Check sheet for the drawn part. Datum: minimum x, y, z corner. Units: mm. A direction names the side the tool comes from. Round coordinates to 2 decimals unless told otherwise and drop trailing zeros. Write each loop counter-clockwise with the first axis right and the second up, starting at its lowest first coordinate (ties: lowest second). Pieces come first, ordered by that corner, then holes.
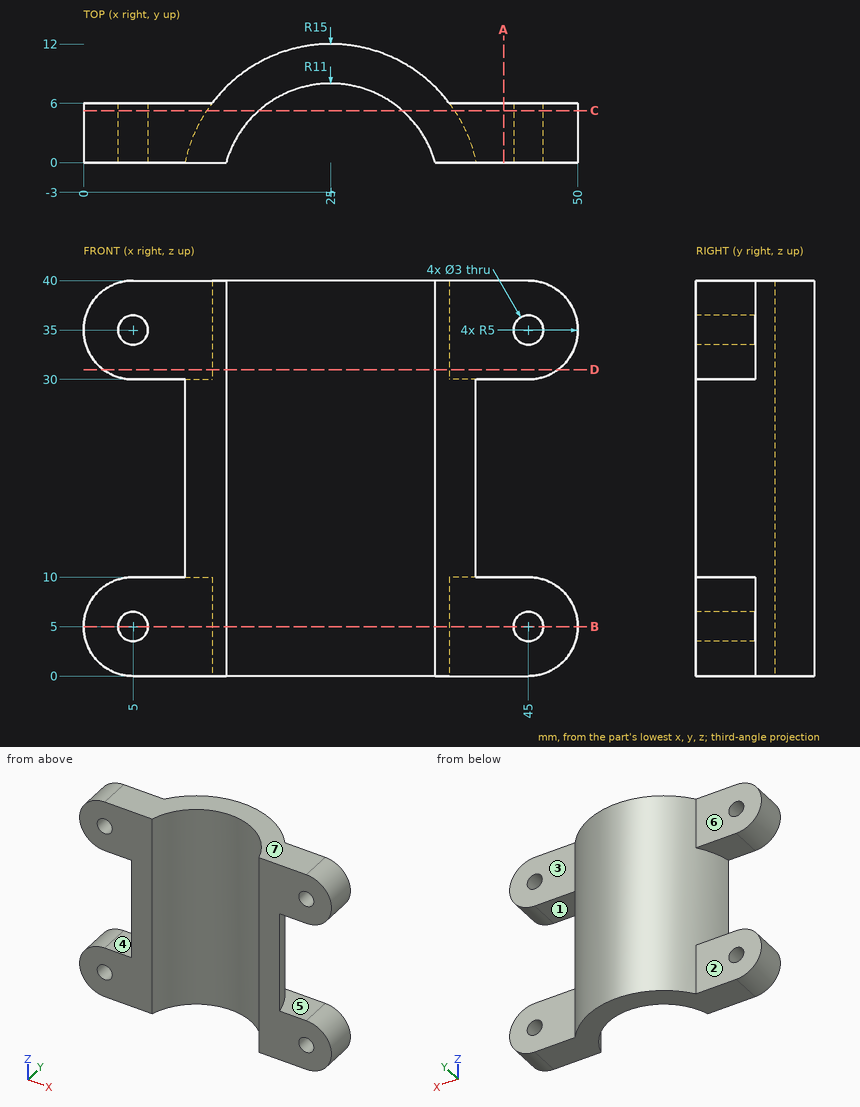
Q1. Depth check by flat-ended pin: P1, Ø4, axis at x = 45, z = 5, coming from the +Y side; P2, Ø1.8, axis at x = 5, z = 35, coming from the +Y side; P3, Ø1, axis at y = 10, z = 6.5, coming from the -X side. Enter the tip coordinate at first touch or a pass-through.
Recorded:
P1: stops at y = 6
P2: passes through
P3: stops at x = 16.71
Q2. Sectioned sample at B-B (z = 5). Enter the section's corners in (x, y).
Recorded:
outline: (0, 0) - (3.5, 0) - (3.5, 6) - (0, 6) - close; (6.5, 0) - (14.42, 0) arc R11 cw to (35.58, 0) - (43.5, 0) - (43.5, 6) - (37, 6) arc R15 ccw to (13, 6) - (6.5, 6) - close; (46.5, 0) - (50, 0) - (50, 6) - (46.5, 6) - close
Q3. Release check for a two-part mould opening along Z. For the marked faces 5, 6 and 7 record: released by +Z, released by -Z, zero draft, split by the parting line, or undercut.
Recorded:
face 5: undercut
face 6: zero draft
face 7: released by +Z
Q4. Tool access check on the marked faces 1, 2, 3 and 4. Record the directions out of +Z, -Z, +X, -X, +Y, -Y that give a thin tool (end or side, any length) a straight path to the whole face; none if there is none.
Recorded:
face 1: +X, +Y
face 2: +Z, -Z, -X, +Y
face 3: +Z, -Z, +X, +Y
face 4: -X, +Y
Q5. Material ranges on line 1 along Z through (x, y) = (5, 4.35); line 2 along X through (y, z) = (3.4, 5); line 3 along Y through (x, z) = (24.5, 21), recorded low to high.
Recorded:
line 1: z = 0 to 3.5, 6.5 to 10, 30 to 33.5, 36.5 to 40
line 2: x = 0 to 3.5, 6.5 to 16.05, 33.95 to 43.5, 46.5 to 50
line 3: y = 7.99 to 11.99
Q6. Sectioned sample at A-A (x = 42.5). Enter the section's corners in (y, z).
Recorded:
outline: (0, 0) - (6, 0) - (6, 10) - (0, 10) - close; (0, 30) - (6, 30) - (6, 40) - (0, 40) - close
Q7. Sectioned sample at C-C (y = 5.25). Enter the section's corners in (x, z).
Recorded:
outline: (5, 0) - (17.72, 0) - (17.72, 40) - (5, 40) arc R5 ccw to (5, 30) - (12.47, 30) - (12.47, 10) - (5, 10) arc R5 ccw to start; (32.28, 0) - (45, 0) arc R5 ccw to (45, 10) - (37.53, 10) - (37.53, 30) - (45, 30) arc R5 ccw to (45, 40) - (32.28, 40) - close; hole circle Ø3 at (5, 5); hole circle Ø3 at (5, 35); hole circle Ø3 at (45, 5); hole circle Ø3 at (45, 35)
Q8. Sectioned sample at D-D (z = 31). Enter the section's corners in (x, y), plus the area to 3 significant figures.
Recorded:
outline: (2, 0) - (14.42, 0) arc R11 cw to (35.58, 0) - (48, 0) - (48, 6) - (37, 6) arc R15 ccw to (13, 6) - (2, 6) - close
area: 252 mm2
